Check sheet for the modelled part. Datum: model origin and axes. Units: mm. A direction names the side the tool comes from. Coordinates: 2 decimals unless noted, no trailing zeros. Loops run counter-clockwise (first coordinate to the right, second up) from the corner with the lowest first, then second, coordinate; pieces in that order, holes last. Notation, with made-up numbers: (11.25, -11) - (68.25, -11) arc R9 cw to (68.25, 2) - close; hole circle Ø3 at (-0.75, 43.5). An arc over 180 degrees is marked (long way). Use a Markdown table: item, result. Add a question column.
1) Sectioned sample at C-C, the plane x = 42.5. Enter the section's corners in (y, z), then the cut area to 3 significant figures.
2) Go/stop test with flat-tipped pins: P1, Ø5, axis at y = -88, z = 14.5, coming from the +X side; P2, Ø12, axis at y = -116, z = 15, coming from the +X side; P3, Ø2, axis at x = 42.5, y = -120, coming from the +Z side. Record where each tip stops, or that it passes through.
3) Thickness scan on line 1 (Y direction, x = 147.5, z = 11.25); line 2 (Y direction, x = 45, z = 16.5); line 3 (Y direction, x = 148.5, z = 2.5). Record the ranges inside material, lowest first.
4) Sectioned sample at A-A, the plane z = 16.75. State how many separate pieces and enclosed holes the cut face has, then the cut area to 3 significant figures.
5) Draft check along Y on faces 1 (the flat face through (146, -36, 20)), 2 (the cylindrical face through (151.315, -38.799, 11.126)), 3 (the cylindrical face through (39.92, -37.635, 11.126)). Enter one of: pulls with the +Y half, pulls with the -Y half, needs draft (parallel to the pull), parting line crosses it, or undercut.
6) Sectioned sample at B-B, the plane y = -120. Enter the section's corners in (x, z).
7) Tool access check on faces 4 (the cylindrical face through (90.381, -78.085, 10.874)), 5 (the flat face through (200, -76, 3)). Record the directions out of +Z, -Z, +X, -X, +Y, -Y that give a thin tool (end or side, any length) a straight path to the whole face; none if there is none.
8) Sectioned sample at D-D, the plane x = 124. Enter the section's corners in (y, z).
from build123d import *

# Parameters (mm, degrees)
ESQUISSE1_W             = 200
ESQUISSE1_H             = 150
BOSS_EXTRU_1_DEPTH      = 2
ESQUISSE2_R             = 6
ESQUISSE2_R_2           = 5
BOSS_EXTRU_3_DEPTH      = 20
ESQUISSE3_W             = 200
ESQUISSE3_H             = 150
ESQUISSE3_W_2           = 196
ESQUISSE3_H_2           = 146
BOSS_EXTRU_4_DEPTH      = 4
ESQUISSE4_R             = 4
ENL_V_MAT_EXTRU_1_DEPTH = 18
ENL_V_START             = 18
ESQUISSE5_R             = 3.5
ENL_V_MAT_EXTRU_4_DEPTH = 18
ESQUISSE6_R             = 3.5
ENL_V_MAT_EXTRU_6_DEPTH = 18
ESQUISSE7_R             = 3.5
ENL_V_MAT_EXTRU_7_DEPTH = 18
ESQUISSE8_R             = 2.5
ENL_V_MAT_EXTRU_8_DEPTH = 18


with BuildPart() as part:
    # Esquisse1 → Boss.-Extru.1 (new body)
    with BuildSketch(Plane.XY):
        with Locations((100, -75)):
            Rectangle(ESQUISSE1_W, ESQUISSE1_H)
    extrude(amount=BOSS_EXTRU_1_DEPTH)

    # Esquisse2 → Boss.-Extru.3 (add)
    with BuildSketch(Plane.XY):
        with Locations(Location((42.5, -120, 0), (0, 0, 180))):
            Circle(ESQUISSE2_R)
        with Locations(Location((42.5, -40, 0), (0, 0, 180))):
            Circle(ESQUISSE2_R)
        with Locations(Location((147.5, -120, 0), (0, 0, 180))):
            Circle(ESQUISSE2_R)
        with Locations(Location((147.5, -40, 0), (0, 0, 180))):
            Circle(ESQUISSE2_R)
        with Locations(Location((95, -80, 0), (0, 0, 180))):
            Circle(ESQUISSE2_R_2)
    extrude(amount=BOSS_EXTRU_3_DEPTH)

    # Esquisse3 → Boss.-Extru.4 (add)
    with BuildSketch(Plane.XY.offset(2)):
        with Locations((100, -75)):
            Rectangle(ESQUISSE3_W, ESQUISSE3_H)
        with Locations((100, -75)):
            Rectangle(ESQUISSE3_W_2, ESQUISSE3_H_2, mode=Mode.SUBTRACT)
    extrude(amount=BOSS_EXTRU_4_DEPTH)

    # Esquisse4 → Enlèv. mat.-Extru.1 (cut)
    with BuildSketch(Plane.XY.offset(20)):
        with Locations((147.5, -40)):
            Circle(ESQUISSE4_R)
    extrude(amount=-ENL_V_MAT_EXTRU_1_DEPTH, mode=Mode.SUBTRACT)

    # Esquisse5 → Enlèv. mat.-Extru.4 (cut)
    with BuildSketch(Plane.XY.offset(2).offset(ENL_V_START)):
        with Locations((42.5, -40)):
            Circle(ESQUISSE5_R)
    extrude(amount=-ENL_V_MAT_EXTRU_4_DEPTH, mode=Mode.SUBTRACT)

    # Esquisse6 → Enlèv. mat.-Extru.6 (cut)
    with BuildSketch(Plane.XY.offset(2).offset(ENL_V_START)):
        with Locations((147.5, -120)):
            Circle(ESQUISSE6_R)
    extrude(amount=-ENL_V_MAT_EXTRU_6_DEPTH, mode=Mode.SUBTRACT)

    # Esquisse7 → Enlèv. mat.-Extru.7 (cut)
    with BuildSketch(Plane.XY.offset(2).offset(ENL_V_START)):
        with Locations((42.5, -120)):
            Circle(ESQUISSE7_R)
    extrude(amount=-ENL_V_MAT_EXTRU_7_DEPTH, mode=Mode.SUBTRACT)

    # Esquisse8 → Enlèv. mat.-Extru.8 (cut)
    with BuildSketch(Plane.XY.offset(2).offset(ENL_V_START)):
        with Locations((95, -80)):
            Circle(ESQUISSE8_R)
    extrude(amount=-ENL_V_MAT_EXTRU_8_DEPTH, mode=Mode.SUBTRACT)


solid = part.part
Solved:
| question | item | result |
|---|---|---|
| 1 | outline | (-150, 0) - (0, 0) - (0, 6) - (-2, 6) - (-2, 2) - (-34, 2) - (-34, 20) - (-36.5, 20) - (-36.5, 2) - (-43.5, 2) - (-43.5, 20) - (-46, 20) - (-46, 2) - (-114, 2) - (-114, 20) - (-116.5, 20) - (-116.5, 2) - (-123.5, 2) - (-123.5, 20) - (-126, 20) - (-126, 2) - (-148, 2) - (-148, 6) - (-150, 6) - close |
| 1 | area | 496 mm2 |
| 2 | P1 | passes through |
| 2 | P2 | stops at x = 153.5 |
| 2 | P3 | stops at z = 2 |
| 3 | line 1 | y = -126 to -123.5, -116.5 to -114, -46 to -44, -36 to -34 |
| 3 | line 2 | y = -125.45 to -122.45, -117.55 to -114.55, -45.45 to -42.45, -37.55 to -34.55 |
| 3 | line 3 | y = -150 to -148, -125.92 to -123.35, -116.65 to -114.08, -45.92 to -43.87, -36.13 to -34.08, -2 to 0 |
| 4 | separate pieces | 5 |
| 4 | enclosed holes | 5 |
| 4 | area | 346 mm2 |
| 5 | face 1 | needs draft |
| 5 | face 2 | undercut |
| 5 | face 3 | undercut |
| 6 | outline | (0, 0) - (200, 0) - (200, 6) - (198, 6) - (198, 2) - (153.5, 2) - (153.5, 20) - (151, 20) - (151, 2) - (144, 2) - (144, 20) - (141.5, 20) - (141.5, 2) - (48.5, 2) - (48.5, 20) - (46, 20) - (46, 2) - (39, 2) - (39, 20) - (36.5, 20) - (36.5, 2) - (2, 2) - (2, 6) - (0, 6) - close |
| 7 | face 4 | +Z |
| 7 | face 5 | +Z, -Z, +X, +Y, -Y |
| 8 | outline | (-150, 0) - (0, 0) - (0, 6) - (-2, 6) - (-2, 2) - (-148, 2) - (-148, 6) - (-150, 6) - close |
